Geometry check sheet. Reference: the model listing, model coordinates, mm. Face numbers are marked on the shaded views. Give positions to 0.01 mm unless a question says otherwise; leave off trailing zeros. Order: outer loops, then holes, each group sorted by start corner. A loop starts at its lowest first (then second) coordinate and runs counter-clockwise, first axis right, second up. Notation, with made-up numbers: M -6,86.5 L 49,86.5 A19 cw 49,110.5 Z; hole C 47.5,69 d1. An arc over 180 degrees is marked long. Answer as a JSON object with one key per item and string values. Group by question number.
from build123d import *

# Parameters (mm, degrees)
SKIZZE1_W                       = 14.5
SKIZZE1_H                       = 2.9
AUFSATZ_LINEAR_AUSTRAGEN1_DEPTH = 1.45
VERRUNDUNG1_RADIUS              = 1.45
VERRUNDUNG1_LENGTH              = 2.9
VERRUNDUNG2_RADIUS              = 1.45
VERRUNDUNG2_LENGTH              = 2.9
SKIZZE2_R                       = 0.25
AUFSATZ_LINEAR_AUSTRAGEN2_DEPTH = 1.1


with BuildPart() as part:
    # Skizze1 → Aufsatz-Linear austragen1 (new, symmetric)
    with BuildSketch(Plane.XY):
        Rectangle(SKIZZE1_W, SKIZZE1_H)
    extrude(amount=AUFSATZ_LINEAR_AUSTRAGEN1_DEPTH, both=True)

    # Verrundung1: full round fillet: the end face becomes a half cylinder, R = half its width
    verrundung1_face = Plane((7.25, 0, 0), x_dir=(0, -1, 0), z_dir=(1, 0, 0))  # on the end face: x along it, z out of the body
    verrundung1_slab = verrundung1_face.offset(-VERRUNDUNG1_RADIUS / 2) * Box(VERRUNDUNG1_LENGTH, 2 * VERRUNDUNG1_RADIUS, VERRUNDUNG1_RADIUS, mode=Mode.PRIVATE)  # the body's end, R deep
    verrundung1_round = Plane((5.8, 0, 0), x_dir=(1, 0, 0), z_dir=(0, -1, 0)) * Cylinder(VERRUNDUNG1_RADIUS, VERRUNDUNG1_LENGTH, mode=Mode.PRIVATE)  # its axis R under the face
    add(verrundung1_slab - verrundung1_round, mode=Mode.SUBTRACT)

    # Verrundung2: full round fillet: the end face becomes a half cylinder, R = half its width
    verrundung2_face = Plane((-7.25, 0, 0), x_dir=(0, 1, 0), z_dir=(-1, 0, 0))  # on the end face: x along it, z out of the body
    verrundung2_slab = verrundung2_face.offset(-VERRUNDUNG2_RADIUS / 2) * Box(VERRUNDUNG2_LENGTH, 2 * VERRUNDUNG2_RADIUS, VERRUNDUNG2_RADIUS, mode=Mode.PRIVATE)  # the body's end, R deep
    verrundung2_round = Plane((-5.8, 0, 0), x_dir=(-1, 0, 0), z_dir=(0, 1, 0)) * Cylinder(VERRUNDUNG2_RADIUS, VERRUNDUNG2_LENGTH, mode=Mode.PRIVATE)  # its axis R under the face
    add(verrundung2_slab - verrundung2_round, mode=Mode.SUBTRACT)

    # Skizze2 → Aufsatz-Linear austragen2 (add)
    with BuildSketch(Plane.XZ.offset(1.45)):
        with Locations(Location((-5.8, 0, 0), (0, 0, 90))):
            Circle(SKIZZE2_R)
        with Locations(Location((5.8, 0, 0), (0, 0, 90))):
            Circle(SKIZZE2_R)
    extrude(amount=AUFSATZ_LINEAR_AUSTRAGEN2_DEPTH)


solid = part.part
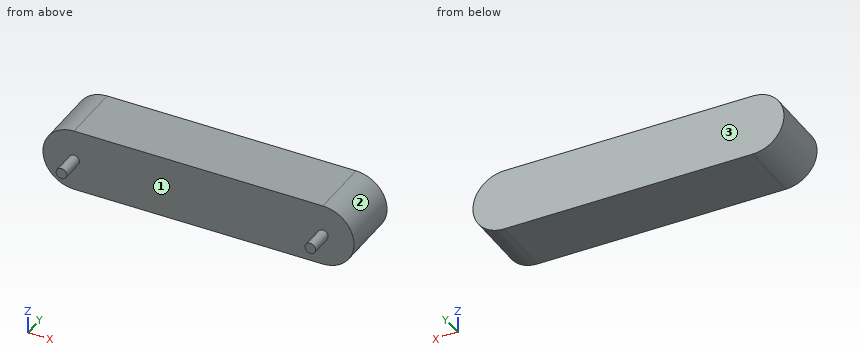
1. Cross-section at D-D (x = -0.5). Record the cut outline in (y, z).
2. Thickness scan on line 1 along Y through (x, z) = (-2.75, -0.45); line 2 along X through (y, z) = (0.7, -0.5); line 3 along X through (y, z) = (-0.05, -1.2). Record the ranges inside material, lowest first. Write a range as [from, to].
3. Cross-section at C-C (y = 1.1). Record the cut outline in (x, z).
4. Cross-section at A-A (y = -1.6). Record the cut outline in (x, z).
5. Depth check by flat-ended pin: pin 1 (0.9 mm diameter, centred on x = 3, z = 0, fed in from -Y); pin 2 (1 mm diameter, centred on y = -1.5, z = 1, fed in from +X). Enter the tip coordinate at first touch or a pass-through.
6. Release check for a two-part mould opening along Y. For the marked faces 1, 2 and 3 record: released by +Y, released by -Y, zero draft, split by the parting line, or undercut.
7. Cross-section at B-B (z = 0). Record the cut outline in (x, y).
Report:
{
 "1": {"outline": "M -1.45,-1.45 L 1.45,-1.45 L 1.45,1.45 L -1.45,1.45 Z"},
 "2": {"line 1": "y = [-1.45, 1.45]", "line 2": "x = [-7.16, 7.16]", "line 3": "x = [-6.61, 6.61]"},
 "3": {"outline": "M -5.8,-1.45 L 5.8,-1.45 A1.45 ccw 5.8,1.45 L -5.8,1.45 A1.45 ccw Z"},
 "4": {"outline": "C -5.8,0 d0.5; C 5.8,0 d0.5"},
 "5": {"pin 1": "stops at y = -1.45", "pin 2": "stops at x = 7.16"},
 "6": {"face 1": "released by -Y", "face 2": "zero draft", "face 3": "released by +Y"},
 "7": {"outline": "M -7.25,-1.45 L -6.05,-1.45 L -6.05,-2.55 L -5.55,-2.55 L -5.55,-1.45 L 5.55,-1.45 L 5.55,-2.55 L 6.05,-2.55 L 6.05,-1.45 L 7.25,-1.45 L 7.25,1.45 L -7.25,1.45 Z"}
}
